from build123d import *

# Parameters (mm, degrees)
F0_R     = 1.75
F0_W     = 5
F0_H     = 3
F0_R_2   = 1.6
F0_W_2   = 20
F0_H_2   = 5
F0_R_3   = 19
F1_DEPTH = 5


with BuildPart() as f1:
    # F0 (on Top) → F1 (new body)
    with BuildSketch(Plane.XY):
        Polygon((15, 100), (0, 100), (0, 65), (5, 65), (5, 60), (0, 60), (0, 40), (5, 40), (5, 35), (0, 35), (0, 0), (15, 0), (15, 5), (20, 5), (20, 0), (40, 0), (40, 5), (45, 5), (45, 0), (125, 0), (125, 5), (130, 5), (130, 0), (150, 0), (150, 5), (155, 5), (155, 0), (170, 0), (170, 10), (162, 10), (162, 25), (170, 25), (170, 35), (165, 35), (165, 40), (170, 40), (170, 60), (165, 60), (165, 65), (170, 65), (170, 100), (155, 100), (155, 95), (150, 95), (150, 100), (130, 100), (130, 95), (125, 95), (125, 100), (45, 100), (45, 95), (40, 95), (40, 100), (20, 100), (20, 95), (15, 95), align=None)
        with Locations((30, 2.5)):
            Circle(F0_R, mode=Mode.SUBTRACT)
        with Locations((140, 2.5)):
            Circle(F0_R, mode=Mode.SUBTRACT)
        with Locations((97.5, 28.5)):
            Rectangle(F0_W, F0_H, mode=Mode.SUBTRACT)
        with Locations((101, 34)):
            Circle(F0_R_2, mode=Mode.SUBTRACT)
        with Locations((140, 27.5)):
            Rectangle(F0_W_2, F0_H_2, mode=Mode.SUBTRACT)
        with Locations((2.5, 50)):
            Circle(F0_R, mode=Mode.SUBTRACT)
        with Locations((69, 66)):
            Circle(F0_R_2, mode=Mode.SUBTRACT)
        with Locations((30, 97.5)):
            Circle(F0_R, mode=Mode.SUBTRACT)
        with Locations((85, 50)):
            Circle(F0_R_3, mode=Mode.SUBTRACT)
        with Locations((167.5, 50)):
            Circle(F0_R, mode=Mode.SUBTRACT)
        with Locations((140, 72.5)):
            Rectangle(F0_W_2, F0_H_2, mode=Mode.SUBTRACT)
        with Locations((140, 97.5)):
            Circle(F0_R, mode=Mode.SUBTRACT)
    extrude(amount=F1_DEPTH)


solid = f1.part
Source: CAD feature listing. Evaluate the final solid. Frame: model axes, mm. A direction names the side the tool comes from. Round coordinates to 2 decimals unless told otherwise and drop trailing zeros. Loops run counter-clockwise (first coordinate to the right, second up) from the corner with the lowest first, then second, coordinate; pieces in that order, holes last. Notation, with made-up numbers: M 87.25,-24 L 115.25,-24 A28 ccw 115.25,0 Z; hole C 78.5,55 d5. An arc over 180 degrees is marked long. Return JSON: item names as keys, results as strings. Group by question number.
1. Section query B-B on x = 85. Output: boundary loops of the cut face in (y, z), and give its area (3 significant figures).
2. Material intervals for line 1 along Y through (x, z) = (2.5, 3); line 2 along Y through (x, z) = (30, 3.65); line 3 along X through (y, z) = (29, 1.1), sorted ascending. Write a range as from..to.
3. Pin query (flat end, axial travel): pin 1 (1.5 mm diameter, centred on x = 152.5, z = 3.5, fed in from -Y); pin 2 (2.5 mm diameter, centred on y = 62, z = 3, fed in from +X); pin 3 (3 mm diameter, centred on x = 140, y = 2.5, fed in from -Z). Return the tip coordinate at first contact, or that it passes through.
4. Section query D-D on x = 167.5. Output: boundary loops of the cut face in (y, z), and give its area (4 significant figures).
5. Section query C-C on y = 50. Output: boundary loops of the cut face in (x, z).
6. Mould query, pull axis X, two halves, no side actions, for faces 5 (the face through (168, 35, 2)), 6 (the face through (155, 98, 2)), 7 (the face through (130, 27, 2)), 8 (the face through (0, 83, 2)). Classes: released by +X, released by -X, zero draft, split by the parting line, or undercut.
7. Reachability of faces 1 (the face through (15, 97, 2)), 2 (the face through (5, 63, 2)), 3 (the face through (17, 5, 2)), 4 (the face through (130, 72, 2)) from +Z, -Z, +X, -X, +Y, -Y: full face, straight path, thin tool, end or side. Return the list, or none.
8. Section query A-A on y = 2.5. Output: boundary loops of the cut face in (x, z), and give its area (3 significant figures).
Checks:
{
 "1": {"outline": "M 0,0 L 31,0 L 31,5 L 0,5 Z; M 69,0 L 100,0 L 100,5 L 69,5 Z", "area": "310 mm²"},
 "2": {"line 1": "y = 0..35, 40..48.25, 51.75..60, 65..100", "line 2": "y = 0..0.75, 4.25..95.75, 99.25..100", "line 3": "x = 0..95, 100..130, 150..170"},
 "3": {"pin 1": "stops at y = 5", "pin 2": "stops at x = 165", "pin 3": "passes through"},
 "4": {"outline": "M 0,0 L 10,0 L 10,5 L 0,5 Z; M 25,0 L 35,0 L 35,5 L 25,5 Z; M 40,0 L 48.25,0 L 48.25,5 L 40,5 Z; M 51.75,0 L 60,0 L 60,5 L 51.75,5 Z; M 65,0 L 100,0 L 100,5 L 65,5 Z", "area": "357.5 mm²"},
 "5": {"outline": "M 0,0 L 0.75,0 L 0.75,5 L 0,5 Z; M 4.25,0 L 66,0 L 66,5 L 4.25,5 Z; M 104,0 L 165.75,0 L 165.75,5 L 104,5 Z; M 169.25,0 L 170,0 L 170,5 L 169.25,5 Z"},
 "6": {"face 5": "zero draft", "face 6": "undercut", "face 7": "undercut", "face 8": "released by -X"},
 "7": {"face 1": "+Z, -Z, +Y", "face 2": "+Z, -Z, -X", "face 3": "+Z, -Z, -Y", "face 4": "+Z, -Z"},
 "8": {"outline": "M 0,0 L 15,0 L 15,5 L 0,5 Z; M 20,0 L 28.25,0 L 28.25,5 L 20,5 Z; M 31.75,0 L 40,0 L 40,5 L 31.75,5 Z; M 45,0 L 125,0 L 125,5 L 45,5 Z; M 130,0 L 138.25,0 L 138.25,5 L 130,5 Z; M 141.75,0 L 150,0 L 150,5 L 141.75,5 Z; M 155,0 L 170,0 L 170,5 L 155,5 Z", "area": "715 mm²"}
}
